For this review, take the finished solid that the model builds, in its own axes (mm). Round coordinates to 2 decimals unless told otherwise and drop trailing zeros. Order: outer loops, then holes, each group sorted by start corner. A loop starts at its lowest first (then second) coordinate and runs counter-clockwise, first axis right, second up. Notation, with made-up numbers: (67, 75) -> (76, 75) arc R26 ccw to (76, 93) -> close; hole circle Ø6 at (-20.75, 44.25). An arc over 180 degrees is marked (long way). Use a Markdown table: item, result. Add a question column.
1) Wall thickness on line 1 along Y through (x, z) = (38, 1.1); line 2 along X through (y, z) = (-1, 1.65); line 3 along X through (y, z) = (-1, 1.7): over which ranges is each line inside the solid? List them lowest first. Write a range as [from, to].
2) Draft analysis for pull direction Y (two halves, no side actions). For faces 1 (the face through (19, -4, 1)), 2 (the face through (52, 0, 1)), 3 (the face through (36.82, 1.08, 0.79)), state which applies: pulls with the +Y half, pulls with the -Y half, needs draft (parallel to the pull), parting line crosses it, or undercut.
3) Consider section A-A (y = 0). State the section outline as (x, z) points, plus the area to 3 significant figures.
4) Consider section B-B (z = 2.2). State the section outline as (x, y) points.
5) Consider section C-C (x = 38). State the section outline as (y, z) points, plus the area to 3 significant figures.
6) Clearance check with a flat-ended pin moving along its axis: P1, Ø3.5, axis at x = 48, y = 0, coming from the -Z side. State where the tip first meets the part, or that it passes through.
```python
from build123d import *

# Parameters (mm, degrees)
SKETCH_1_R      = 1.6
EXTRUDE_1_DEPTH = 3
CHAMFER_1_SIZE  = 1.4


with BuildPart() as part:
    # 草图1 → 凸台-拉伸1 (new body)
    with BuildSketch(Plane.XY):
        with BuildLine():
            Line((-10, 4), (48, 4))
            ThreePointArc((48, 4), (52, 0), (48, -4))
            Line((48, -4), (-10, -4))
            ThreePointArc((-10, -4), (-14, 0), (-10, 4))
        make_face()
        Circle(SKETCH_1_R, mode=Mode.SUBTRACT)
        with Locations((38, 0)):
            Circle(SKETCH_1_R, mode=Mode.SUBTRACT)
        with Locations((-10, 0)):
            Circle(SKETCH_1_R, mode=Mode.SUBTRACT)
        with Locations((48, 0)):
            Circle(SKETCH_1_R, mode=Mode.SUBTRACT)
    extrude(amount=EXTRUDE_1_DEPTH)

    # 倒角1
    chamfer_1_edges = [part.edges().sort_by_distance(p)[0] for p in [
        (-1.6, 0, 3),
        (-11.6, 0, 0),
        (46.4, 0, 0),
        (36.4, 0, 3),
    ]]
    chamfer(chamfer_1_edges, length=CHAMFER_1_SIZE)


solid = part.part
```
Results list:
| question | item | result |
|---|---|---|
| 1 | line 1 | [-4, -1.6], [1.6, 4] |
| 1 | line 2 | [-13.87, -11.25], [-8.75, -1.31], [1.31, 36.69], [39.31, 46.75], [49.25, 51.87] |
| 1 | line 3 | [-13.87, -11.25], [-8.75, -1.37], [1.37, 36.63], [39.37, 46.75], [49.25, 51.87] |
| 2 | face 1 | pulls with the -Y half |
| 2 | face 2 | parting line crosses it |
| 2 | face 3 | undercut |
| 3 | outline | (-14, 0) -> (-13, 0) -> (-11.6, 1.4) -> (-11.6, 3) -> (-14, 3) -> close; (-8.4, 1.4) -> (-7, 0) -> (-1.6, 0) -> (-1.6, 1.6) -> (-3, 3) -> (-8.4, 3) -> close; (1.6, 0) -> (36.4, 0) -> (36.4, 1.6) -> (35, 3) -> (3, 3) -> (1.6, 1.6) -> close; (39.6, 0) -> (45, 0) -> (46.4, 1.4) -> (46.4, 3) -> (41, 3) -> (39.6, 1.6) -> close; (49.6, 1.4) -> (51, 0) -> (52, 0) -> (52, 3) -> (49.6, 3) -> close |
| 3 | area | 152 mm2 |
| 4 | outline | (-10, -4) -> (48, -4) arc R4 ccw to (48, 4) -> (-10, 4) arc R4 ccw to start; hole circle Ø3.2 at (-10, 0); hole circle Ø4.4 at (0, 0); hole circle Ø4.4 at (38, 0); hole circle Ø3.2 at (48, 0) |
| 5 | outline | (-4, 0) -> (-1.6, 0) -> (-1.6, 1.6) -> (-3, 3) -> (-4, 3) -> close; (1.6, 0) -> (4, 0) -> (4, 3) -> (3, 3) -> (1.6, 1.6) -> close |
| 5 | area | 12.4 mm2 |
| 6 | P1 | z = 1.25 |
